Geometry: final body of the model. Coordinates: model frame, mm. Give positions to 0.01 mm unless a question says otherwise; leave off trailing zeros. Order: outer loops, then holes, each group sorted by start corner. A loop starts at its lowest first (then second) coordinate and runs counter-clockwise, first axis right, second up. Notation, with made-up numbers: (63.5, 67.25) -> (111.5, 67.25) arc R16 ccw to (111.5, 81.25) -> close; hole circle Ø11 at (-17, 50). An arc over 180 degrees is marked (long way). Answer in a Markdown table with one row per item. Add a question column.
Q1. Contact query for flat-ended pins moving along their axis: P1, Ø1, axis at x = -15, y = -6.5, coming from the -Z side; P2, Ø1.5, axis at y = -2.5, z = 9, coming from the -X side; P3, Ø1, axis at y = -8, z = 13, coming from the +X side; P4, Ø1.5, axis at y = 7, z = 6.5, coming from the +X side. Output: stop coordinate, or through.
Q2. Line query: line 1 along X through (y, z) = (17, 5.75); line 2 along Y through (x, z) = (0, 0.75); line 3 along X through (y, z) = (-14, 11). Output: solid intervals per line, ascending. Write a range as from..to.
Q3. Cut plane C-C on x = 14. Return the cut outline in (y, z), and give its area (3 significant figures).
Q4. Cut plane B-B on y = -10.5. Return the cut outline in (x, z), and give its area (3 significant figures).
Q5. Cut plane A-A on z = 6.5. Return the cut outline in (x, y).
Q6. Pull-direction query (X, two-part tool) for faces 1 (the face through (-18.5, -7.6, 7.4)), 2 (the face through (-11.232, 11.112, 7.395)), 3 (the face through (11.232, -11.112, 7.395)), 4 (the face through (7.7, 18.46, 7.4)); classes: +X half, -X half, draft (parallel to the pull), parting line (faces both ways), or undercut.
Q7. Cut plane D-D on y = 15. Return the cut outline in (x, z).
from build123d import *

# Parameters (mm, degrees)
CYLINDER002_R     = 4
CYLINDER002_DEPTH = 15
CYLINDER003_R     = 4
CYLINDER003_DEPTH = 15
CYLINDER004_R     = 4
CYLINDER004_DEPTH = 15
CYLINDER005_R     = 4
CYLINDER005_DEPTH = 15
CYLINDER007_R     = 4
CYLINDER007_DEPTH = 15
CYLINDER006_R     = 4
CYLINDER006_DEPTH = 15
CYLINDER008_R     = 4
CYLINDER008_DEPTH = 15
CYLINDER001_R     = 4
CYLINDER001_DEPTH = 15
CYLINDER_R        = 20
CYLINDER_DEPTH    = 15


with BuildPart() as cylinder002:
    # Cylinder002 → Cylinder002 (new body)
    with BuildSketch(Plane(origin=(0, 20, 0), x_dir=(1, 0, 0), z_dir=(0, 0, 1))):
        Circle(CYLINDER002_R)
    extrude(amount=CYLINDER002_DEPTH)


with BuildPart() as cylinder003:
    # Cylinder003 → Cylinder003 (new body)
    with BuildSketch(Plane(origin=(-20, 0, 0), x_dir=(1, 0, 0), z_dir=(0, 0, 1))):
        Circle(CYLINDER003_R)
    extrude(amount=CYLINDER003_DEPTH)


with BuildPart() as cylinder004:
    # Cylinder004 → Cylinder004 (new body)
    with BuildSketch(Plane(origin=(0, -20, 0), x_dir=(1, 0, 0), z_dir=(0, 0, 1))):
        Circle(CYLINDER004_R)
    extrude(amount=CYLINDER004_DEPTH)


with BuildPart() as cylinder005:
    # Cylinder005 → Cylinder005 (new body)
    with BuildSketch(Plane(origin=(14, -14, 0), x_dir=(1, 0, 0), z_dir=(0, 0, 1))):
        Circle(CYLINDER005_R)
    extrude(amount=CYLINDER005_DEPTH)


with BuildPart() as cylinder007:
    # Cylinder007 → Cylinder007 (new body)
    with BuildSketch(Plane(origin=(-14, -14, 0), x_dir=(1, 0, 0), z_dir=(0, 0, 1))):
        Circle(CYLINDER007_R)
    extrude(amount=CYLINDER007_DEPTH)


with BuildPart() as cylinder006:
    # Cylinder006 → Cylinder006 (new body)
    with BuildSketch(Plane(origin=(-14, 14, 0), x_dir=(1, 0, 0), z_dir=(0, 0, 1))):
        Circle(CYLINDER006_R)
    extrude(amount=CYLINDER006_DEPTH)


with BuildPart() as cylinder008:
    # Cylinder008 → Cylinder008 (new body)
    with BuildSketch(Plane(origin=(14, 14, 0), x_dir=(1, 0, 0), z_dir=(0, 0, 1))):
        Circle(CYLINDER008_R)
    extrude(amount=CYLINDER008_DEPTH)


with BuildPart() as cylinder001:
    # Cylinder001 → Cylinder001 (new body)
    with BuildSketch(Plane(origin=(20, 0, 0), x_dir=(1, 0, 0), z_dir=(0, 0, 1))):
        Circle(CYLINDER001_R)
    extrude(amount=CYLINDER001_DEPTH)


with BuildPart() as cut007:
    # Cylinder → Cylinder (new body)
    with BuildSketch(Plane.XY):
        Circle(CYLINDER_R)
    extrude(amount=CYLINDER_DEPTH)

    # Cut: cut Cylinder001
    add(cylinder001.part, mode=Mode.SUBTRACT)

    # Cut001: cut Cylinder008
    add(cylinder008.part, mode=Mode.SUBTRACT)

    # Cut002: cut Cylinder006
    add(cylinder006.part, mode=Mode.SUBTRACT)

    # Cut003: cut Cylinder007
    add(cylinder007.part, mode=Mode.SUBTRACT)

    # Cut004: cut Cylinder005
    add(cylinder005.part, mode=Mode.SUBTRACT)

    # Cut005: cut Cylinder004
    add(cylinder004.part, mode=Mode.SUBTRACT)

    # Cut006: cut Cylinder003
    add(cylinder003.part, mode=Mode.SUBTRACT)

    # Cut007: cut Cylinder002
    add(cylinder002.part, mode=Mode.SUBTRACT)


solid = cut007.part
Completed:
| question | item | result |
|---|---|---|
| 1 | P1 | stops at z = 0 |
| 1 | P2 | stops at x = -17.67 |
| 1 | P3 | stops at x = 18.54 |
| 1 | P4 | stops at x = 19 |
| 2 | line 1 | x = -10.54..-2.65, 2.65..10.54 |
| 2 | line 2 | y = -16..16 |
| 2 | line 3 | x = -10..10 |
| 3 | outline | (-10, 0) -> (10, 0) -> (10, 15) -> (-10, 15) -> close |
| 3 | area | 300 mm² |
| 4 | outline | (-17.02, 0) -> (-15.94, 0) -> (-15.94, 15) -> (-17.02, 15) -> close; (-12.06, 0) -> (12.06, 0) -> (12.06, 15) -> (-12.06, 15) -> close; (15.94, 0) -> (17.02, 0) -> (17.02, 15) -> (15.94, 15) -> close |
| 4 | area | 394 mm² |
| 5 | outline | (-19.6, -3.98) arc R20 ccw to (-16.68, -11.03) arc R4 cw to (-11.03, -16.68) arc R20 ccw to (-3.98, -19.6) arc R4 cw to (3.98, -19.6) arc R20 ccw to (11.03, -16.68) arc R4 cw to (16.68, -11.03) arc R20 ccw to (19.6, -3.98) arc R4 cw to (19.6, 3.98) arc R20 ccw to (16.68, 11.03) arc R4 cw to (11.03, 16.68) arc R20 ccw to (3.98, 19.6) arc R4 cw to (-3.98, 19.6) arc R20 ccw to (-11.03, 16.68) arc R4 cw to (-16.68, 11.03) arc R20 ccw to (-19.6, 3.98) arc R4 cw to start |
| 6 | face 1 | -X half |
| 6 | face 2 | undercut |
| 6 | face 3 | undercut |
| 6 | face 4 | +X half |
| 7 | outline | (-10.13, 0) -> (10.13, 0) -> (10.13, 15) -> (-10.13, 15) -> close |
